from build123d import *

# Parameters (mm, degrees)
BOSS_EXTRUDE1_DEPTH = 2.4
SKETCH2_W           = 33.15
SKETCH2_H           = 36
SKETCH2_R           = 11.75
SKETCH2_R_2         = 0.822021887
SKETCH2_R_3         = 0.927108541
BOSS_EXTRUDE2_DEPTH = 2.33
CHAMFER1_SIZE       = 1.2
CHAMFER1_SIZE2      = 2.078460969
SKETCH3_R           = 0.762
CUT_EXTRUDE1_DEPTH  = 5.8
SKETCH4_W           = 4.73
SKETCH4_H           = 36
BOSS_EXTRUDE3_DEPTH = 1
CHAMFER2_SIZE       = 1.2


with BuildPart() as part:
    # Sketch1 → Boss-Extrude1 (new body)
    with BuildSketch(Plane.XY):
        Polygon((-16.575, -18), (16.575, -18), (16.575, -13.05), (-14.975, -13.05), (-14.975, 13.05), (16.575, 13.05), (16.575, 18), (-16.575, 18), align=None)
    extrude(amount=BOSS_EXTRUDE1_DEPTH)

    # Sketch2 → Boss-Extrude2 (add)
    with BuildSketch(Plane.XY.offset(2.4)):
        Rectangle(SKETCH2_W, SKETCH2_H)
        with Locations((0.965, 0)):
            Circle(SKETCH2_R, mode=Mode.SUBTRACT)
        with Locations((13.452978113, 10.377978113)):
            Circle(SKETCH2_R_2, mode=Mode.SUBTRACT)
        with Locations((-11.747891459, -10.272891459)):
            Circle(SKETCH2_R_3, mode=Mode.SUBTRACT)
    extrude(amount=BOSS_EXTRUDE2_DEPTH)

    # Chamfer1
    chamfer1_edges = [part.edges().sort_by_distance(p)[0] for p in [
        (12.630956227, 10.377978113, 4.73),
        (-12.675, -10.272891459, 4.73),
    ]]
    chamfer1_side = [part.faces().sort_by_distance(p)[0] for p in [
        (0, 17.510620546, 4.73),
    ]]
    chamfer(chamfer1_edges, length=CHAMFER1_SIZE, length2=CHAMFER1_SIZE2, reference=chamfer1_side[0])

    # Sketch3 → Cut-Extrude1 (cut)
    with BuildSketch(Plane.XY.offset(4.73)):
        with Locations((-15.575, 16)):
            Circle(SKETCH3_R)
        with Locations(Location((11.575, 16, 0), (0, 0, 180))):
            Circle(SKETCH3_R)
        with Locations((-15.575, -14)):
            Circle(SKETCH3_R)
        with Locations(Location((15.075, -14, 0), (0, 0, 180))):
            Circle(SKETCH3_R)
    extrude(amount=-CUT_EXTRUDE1_DEPTH, mode=Mode.SUBTRACT)

    # Sketch4 → Boss-Extrude3 (add)
    with BuildSketch(Plane.ZY.offset(16.575)):
        with Locations((2.365, 0)):
            Rectangle(SKETCH4_W, SKETCH4_H)
    extrude(amount=BOSS_EXTRUDE3_DEPTH)

    # Chamfer2
    # the kernel refuses this chamfer: 1.2 mm, written as the material it takes off along each edge
    with BuildSketch(Plane(origin=(15.075, -14, 4.73), x_dir=(-1, 0, 0), z_dir=(0, 1, 0))) as chamfer2_piece_1:
        Polygon((0.762 + CHAMFER2_SIZE, 0), (0.762, -CHAMFER2_SIZE), (0.762, 0), align=None)
    revolve(axis=Axis((15.075, -14, 4.73), (0, 0, 1)), mode=Mode.SUBTRACT)
    with BuildSketch(Plane(origin=(-15.575, -14, 4.73), x_dir=(1, 0, 0), z_dir=(0, -1, 0))) as chamfer2_piece_2:
        Polygon((0.762 + CHAMFER2_SIZE, 0), (0.762, -CHAMFER2_SIZE), (0.762, 0), align=None)
    revolve(axis=Axis((-15.575, -14, 4.73), (0, 0, 1)), mode=Mode.SUBTRACT)
    with BuildSketch(Plane(origin=(11.575, 16, 4.73), x_dir=(-1, 0, 0), z_dir=(0, 1, 0))) as chamfer2_piece_3:
        Polygon((0.762 + CHAMFER2_SIZE, 0), (0.762, -CHAMFER2_SIZE), (0.762, 0), align=None)
    revolve(axis=Axis((11.575, 16, 4.73), (0, 0, 1)), mode=Mode.SUBTRACT)
    with BuildSketch(Plane(origin=(-15.575, 16, 4.73), x_dir=(1, 0, 0), z_dir=(0, -1, 0))) as chamfer2_piece_4:
        Polygon((0.762 + CHAMFER2_SIZE, 0), (0.762, -CHAMFER2_SIZE), (0.762, 0), align=None)
    revolve(axis=Axis((-15.575, 16, 4.73), (0, 0, 1)), mode=Mode.SUBTRACT)


solid = part.part
Build history of the part. All positions in model axes, mm. A direction names the side the tool comes from. Give positions to 0.01 mm unless a question says otherwise; leave off trailing zeros. Order: outer loops, then holes, each group sorted by start corner. A loop starts at its lowest first (then second) coordinate and runs counter-clockwise, first axis right, second up. Notation, with made-up numbers: M 70.5,-14 L 116.5,-14 A30 cw 116.5,23 Z; hole C 71.25,88 d11. An arc over 180 degrees is marked long. Put each result on its own line as item: value.
Item 1: Probe line 1 (X direction, y = -8.5, z = 4.4) (1 decimal); line 2 (Y direction, x = -14.5, z = 1.4); line 3 (Z direction, x = -13.5, y = 9). List the from-to ranges inside material, lowest first. Write a range as [from, to].
From the geometry:
line 1: x = [-17.6, -12.5], [-11, -7.1], [9.1, 16.6]
line 2: y = [-18, -13.05], [13.05, 18]
line 3: z = [2.4, 4.73]
Item 2: 3-axis set-ups, long thin cutter, end or side, ignore diameter. For faces 1 (the flat face through (-14.975, 0, 1)), 2 (the flat face through (16.575, 0, 3)): which of +Z, -Z, +X, -X, +Y, -Y reach the whole face in a straight line?
From the geometry:
face 1: -Z, +X
face 2: +Z, -Z, +X, +Y, -Y
Item 3: Slice it at A-A, the plane y = 0. Write the cut outline in (x, z) (3 decimals), plus the area to 3 significant figures.
From the geometry:
outline: M -17.575,0 L -14.975,0 L -14.975,2.4 L -10.785,2.4 L -10.785,4.73 L -17.575,4.73 Z; M 12.715,2.4 L 16.575,2.4 L 16.575,4.73 L 12.715,4.73 Z
area: 31.1 mm2
Item 4: Slice it at B-B, the plane y = 16. Write the cut outline in (x, z) (3 decimals).
From the geometry:
outline: M -17.575,0 L -16.337,0 L -16.337,3.53 L -17.537,4.73 L -17.575,4.73 Z; M -14.813,0 L 10.813,0 L 10.813,3.53 L 9.613,4.73 L -13.613,4.73 L -14.813,3.53 Z; M 12.337,0 L 16.575,0 L 16.575,4.73 L 13.537,4.73 L 12.337,3.53 Z
Item 5: Slice it at D-D, the plane y = 6. Write the cut outline in (x, z) (3 decimals), plus the area to 3 significant figures.
From the geometry:
outline: M -17.575,0 L -14.975,0 L -14.975,2.4 L -9.138,2.4 L -9.138,4.73 L -17.575,4.73 Z; M 11.068,2.4 L 16.575,2.4 L 16.575,4.73 L 11.068,4.73 Z
area: 38.7 mm2
Item 6: Flat gauge pins, fed straight in: pin 1 Ø1.4 at (x, y) = (-15.575, 16) entering from -Z; pin 2 Ø1.5 at (y, z) = (-7, 1.5) entering from +X (3 decimals). Where does each tip first touch, or does it go through?
From the geometry:
pin 1: passes through
pin 2: stops at x = -14.975
Item 7: Slice it at C-C, the plane x = 0. Write the cut outline in (y, z).
From the geometry:
outline: M -18,0 L -13.05,0 L -13.05,2.4 L -11.71,2.4 L -11.71,4.73 L -18,4.73 Z; M 11.71,2.4 L 13.05,2.4 L 13.05,0 L 18,0 L 18,4.73 L 11.71,4.73 Z
Item 8: Two-plate mould, pull along Y, no slides. Class faces 3 (the flat face through (0, -18, 2)), 4 (the cylindrical face through (-0.56, 11.65, 3.55)), 5 (the flat face through (-16, 0, 0)), 6 (the cylindrical face through (15.836, -14.034, 1.79)): +Y half, -Y half, draft (parallel to the pull), parting line (faces both ways), or undercut.
From the geometry:
face 3: -Y half
face 4: undercut
face 5: draft
face 6: undercut
